from build123d import *

# Parameters (mm, degrees)
ESQUISSE1_R                  = 10
ESQUISSE1_W                  = 6.1
ESQUISSE1_H                  = 6.1
BOSS_EXTRU_1_DEPTH           = 5
ESQUISSE2_R                  = 1.8
ENL_V_MAT_EXTRU_1_DEPTH      = 1
ENL_V_MAT_EXTRU_1_DEPTH_BACK = 6
CHANFREIN1_SIZE              = 1


with BuildPart() as part:
    # Esquisse1 → Boss.-Extru.1 (new body)
    with BuildSketch(Plane.XY):
        Circle(ESQUISSE1_R)
        Rectangle(ESQUISSE1_W, ESQUISSE1_H, mode=Mode.SUBTRACT)
    extrude(amount=BOSS_EXTRU_1_DEPTH)

    # Esquisse2 → Enlèv. mat.-Extru.1 (cut, two sides)
    with BuildSketch(Plane.XY.offset(5)) as enl_v_mat_extru_1_sk:
        with Locations((0, 7)):
            Circle(ESQUISSE2_R)
        with Locations((7, 0)):
            Circle(ESQUISSE2_R)
        with Locations((0, -7)):
            Circle(ESQUISSE2_R)
        with Locations((-7, 0)):
            Circle(ESQUISSE2_R)
    extrude(amount=ENL_V_MAT_EXTRU_1_DEPTH, mode=Mode.SUBTRACT)
    extrude(enl_v_mat_extru_1_sk.sketch, amount=-ENL_V_MAT_EXTRU_1_DEPTH_BACK, mode=Mode.SUBTRACT)

    # Chanfrein1
    chanfrein1_edges = [part.edges().sort_by_distance(p)[0] for p in [
        (3.05, -3.05, 2.5),
        (3.05, 3.05, 2.5),
        (-3.05, 3.05, 2.5),
        (-3.05, -3.05, 2.5),
    ]]
    chamfer(chanfrein1_edges, length=CHANFREIN1_SIZE)


solid = part.part
Work out the finished part from the listing and answer in its coordinate system (mm). A direction names the side the tool comes from. Coordinates: 2 decimals unless noted, no trailing zeros. Order: outer loops, then holes, each group sorted by start corner. A loop starts at its lowest first (then second) coordinate and runs counter-clockwise, first axis right, second up. Notation, with made-up numbers: (68.25, 6.25) - (77.25, 6.25) arc R7 ccw to (77.25, 18.25) - close; hole circle Ø11 at (25.25, 69). An arc over 180 degrees is marked (long way). Put each result on its own line as item: value. Start each with the question number.
1) Find section D-D (y = -7). Give the vertices of the cut face in (x, z), plus the area to 3 significant figures.
2) For faces 4 (the flat face through (-2.6, -2.5, 2.5)), 5 (the flat face through (4, 0, 5)), determine the directions among +Z, -Z, +X, -X, +Y, -Y from which every point of the face is accessible in a straight line to the end or side of a thin tool.
3) Find the intervals of material crossed by line 1 (Y direction, x = 0, z = 2.1); line 2 (Y direction, x = 1.25, z = 0.4); line 3 (X direction, y = -0.5, z = 2.1), in increasing order. Write a range as from..to.
4) Find section C-C (z = 0.9). Give the vertices of the cut face in (x, y), plus the area to 3 significant figures.
5) For a pull along Y with two mould halves and no side action, classify faces 1 (the flat face through (-2.5, 2.6, 2.5)), 2 (the flat face through (4, 0, 0)), 3 (the cylindrical face through (-2.17, -9.76, 2.46)) as released by +Y, released by -Y, zero draft, split by the parting line, or undercut.
6) Find section A-A (y = 0). Give the vertices of the cut face in (x, z).
7) Flat-ended cylindrical pins translate along their axes: pin 1 (1.5 mm diameter, centred on x = 4.5, z = 3, fed in from +Y); pin 2 (1.5 mm diameter, centred on x = -7, z = 2, fed in from +Y); pin 3 (3 mm diameter, centred on y = 3, z = 1.5, fed in from -X); pin 4 (3 mm diameter, centred on x = 0, y = 7, fed in from +Z). Find the tip coordinate at first contact, or state that the pin passes through.
Results list:
1. outline: (-7.14, 0) - (-1.8, 0) - (-1.8, 5) - (-7.14, 5) - close; (1.8, 0) - (7.14, 0) - (7.14, 5) - (1.8, 5) - close
1. area: 53.4 mm^2
2. face 4: +Z, -Z
2. face 5: +Z, +X, -X, +Y, -Y
3. line 1: y = -10..-8.8, -5.2..-3.05, 3.05..5.2, 8.8..10
3. line 2: y = -9.92..-8.3, -5.7..-3.05, 3.05..5.7, 8.3..9.92
3. line 3: x = -9.99..-8.73, -5.27..-3.05, 3.05..5.27, 8.73..9.99
4. outline: circle Ø20 at (0, 0); hole circle Ø3.6 at (-7, 0); hole (-3.05, -2.05) - (-2.05, -3.05) - (2.05, -3.05) - (3.05, -2.05) - (3.05, 2.05) - (2.05, 3.05) - (-2.05, 3.05) - (-3.05, 2.05) - close; hole circle Ø3.6 at (0, -7); hole circle Ø3.6 at (0, 7); hole circle Ø3.6 at (7, 0)
4. area: 238 mm^2
5. face 1: undercut
5. face 2: zero draft
5. face 3: split by the parting line
6. outline: (-10, 0) - (-8.8, 0) - (-8.8, 5) - (-10, 5) - close; (-5.2, 0) - (-3.05, 0) - (-3.05, 5) - (-5.2, 5) - close; (3.05, 0) - (5.2, 0) - (5.2, 5) - (3.05, 5) - close; (8.8, 0) - (10, 0) - (10, 5) - (8.8, 5) - close
7. pin 1: stops at y = 9.27
7. pin 2: stops at y = 7.81
7. pin 3: stops at x = -9.89
7. pin 4: passes through
